from build123d import *

# Parameters (mm, degrees)
ESQUISSE1_R             = 1.5
ESQUISSE1_W             = 30
ESQUISSE1_H             = 6
BOSS_EXTRU_3_DEPTH      = 6
ESQUISSE4_W             = 6
ESQUISSE4_H             = 28
ESQUISSE4_H_2           = 85
ESQUISSE4_H_3           = 51
ESQUISSE4_H_4           = 21
ENL_V_MAT_EXTRU_2_DEPTH = 6
ESQUISSE5_R             = 1.5
ENL_V_MAT_EXTRU_3_DEPTH = 9
ENL_V_START             = -3
ESQUISSE6_R             = 1.5
ENL_V_MAT_EXTRU_6_DEPTH = 3
ESQUISSE7_W             = 20
ESQUISSE7_H             = 6
ENL_V_MAT_EXTRU_7_DEPTH = 10
ENL_V_MAT_EXTRU_8_DEPTH = 6
ESQUISSE9_R             = 1.5
ESQUISSE9_W             = 30
ESQUISSE9_H             = 6
ENL_V_MAT_EXTRU_9_DEPTH = 6


with BuildPart() as part:
    # Esquisse1 → Boss.-Extru.3 (new body)
    with BuildSketch(Plane.XY):
        Polygon((19.996437878, 165.487179487), (-0.003562122, 165.487179487), (-0.003562122, -184.512820513), (139.996437878, -184.512820513), (139.996437878, 165.487179487), (119.996437878, 165.487179487), (119.996437878, 105.487179487), (19.996437878, 105.487179487), align=None)
        with Locations((22.996437878, -25.512820513)):
            Circle(ESQUISSE1_R, mode=Mode.SUBTRACT)
        with Locations((69.996437878, -25.512820513)):
            Rectangle(ESQUISSE1_W, ESQUISSE1_H, mode=Mode.SUBTRACT)
        with Locations((116.996437878, -25.512820513)):
            Circle(ESQUISSE1_R, mode=Mode.SUBTRACT)
        with Locations((14.996437878, 162.487179487)):
            Circle(ESQUISSE1_R, mode=Mode.SUBTRACT)
        with Locations((58.496437878, 95.487179487)):
            Circle(ESQUISSE1_R, mode=Mode.SUBTRACT)
        with Locations((81.496437878, 95.487179487)):
            Circle(ESQUISSE1_R, mode=Mode.SUBTRACT)
        with Locations((124.996437878, 162.487179487)):
            Circle(ESQUISSE1_R, mode=Mode.SUBTRACT)
    extrude(amount=BOSS_EXTRU_3_DEPTH)

    # Esquisse4 → Enlèv. mat.-Extru.2 (cut)
    with BuildSketch(Plane.XY):
        with Locations((2.996437878, 151.487179487)):
            Rectangle(ESQUISSE4_W, ESQUISSE4_H)
        with Locations((2.996437878, 64.987179487)):
            Rectangle(ESQUISSE4_W, ESQUISSE4_H_2)
        with Locations((2.996437878, -33.012820513)):
            Rectangle(ESQUISSE4_W, ESQUISSE4_H_3)
        with Locations((136.996437878, -18.012820513)):
            Rectangle(ESQUISSE4_W, ESQUISSE4_H_4)
        with Locations((136.996437878, 64.987179487)):
            Rectangle(ESQUISSE4_W, ESQUISSE4_H_2)
        with Locations((136.996437878, 151.487179487)):
            Rectangle(ESQUISSE4_W, ESQUISSE4_H)
    extrude(amount=ENL_V_MAT_EXTRU_2_DEPTH, mode=Mode.SUBTRACT)

    # Esquisse5 → Enlèv. mat.-Extru.3 (cut)
    with BuildSketch(Plane(origin=(0, 0, 0), x_dir=(0, 0, -1), z_dir=(1, 0, 0))):
        with Locations(Location((-3, -30.012820513, 0), (0, 0, 270))):
            Circle(ESQUISSE5_R)
        with Locations((-3, -0.012820513)):
            Circle(ESQUISSE5_R)
        with Locations(Location((-3, 90.487179487, 0), (0, 0, 270))):
            Circle(ESQUISSE5_R)
        with Locations((-3, 120.487179487)):
            Circle(ESQUISSE5_R)
    extrude(amount=ENL_V_MAT_EXTRU_3_DEPTH, mode=Mode.SUBTRACT)

    # Esquisse6 → Enlèv. mat.-Extru.6 (cut)
    with BuildSketch(Plane(origin=(133.996437878, 0, 0), x_dir=(0, 0, -1), z_dir=(1, 0, 0)).offset(ENL_V_START)):
        with Locations(Location((-3, 90.487179487, 0), (0, 0, 270))):
            Circle(ESQUISSE6_R)
        with Locations(Location((-3, 44.987179487, 0), (0, 0, 90))):
            Circle(ESQUISSE6_R)
        with Locations((-3, 120.487179487)):
            Circle(ESQUISSE6_R)
    extrude(amount=ENL_V_MAT_EXTRU_6_DEPTH, mode=Mode.SUBTRACT)

    # Esquisse7 → Enlèv. mat.-Extru.7 (cut)
    with BuildSketch(Plane.XY):
        with Locations((129.996437878, -181.512820513)):
            Rectangle(ESQUISSE7_W, ESQUISSE7_H)
        with Locations((89.996437878, -181.512820513)):
            Rectangle(ESQUISSE7_W, ESQUISSE7_H)
    extrude(amount=ENL_V_MAT_EXTRU_7_DEPTH, mode=Mode.SUBTRACT)

    # Esquisse8 → Enlèv. mat.-Extru.8 (cut)
    with BuildSketch(Plane.XY.offset(6)):
        with BuildLine():
            Line((79.996437878, -178.512820513), (79.996437878, -113.512820513))
            ThreePointArc((79.996437878, -113.512820513), (42.996437878, -100.746283227), (5.996437878, -113.512820513))
            Line((5.996437878, -113.512820513), (5.996437878, -58.512820513))
            Line((5.996437878, -58.512820513), (-0.003562122, -58.512820513))
            Line((-0.003562122, -58.512820513), (-0.003562122, -184.512820513))
            Line((-0.003562122, -184.512820513), (79.996437878, -184.512820513))
            Line((79.996437878, -184.512820513), (79.996437878, -178.512820513))
        make_face()
    extrude(amount=-ENL_V_MAT_EXTRU_8_DEPTH, mode=Mode.SUBTRACT)

    # Esquisse9 → Enlèv. mat.-Extru.9 (cut)
    with BuildSketch(Plane.XY.offset(6)):
        with Locations((116.996437878, 30.487179487)):
            Circle(ESQUISSE9_R)
        with Locations((22.996437878, 30.487179487)):
            Circle(ESQUISSE9_R)
        with Locations((69.996437878, 30.487179487)):
            Rectangle(ESQUISSE9_W, ESQUISSE9_H)
    extrude(amount=-ENL_V_MAT_EXTRU_9_DEPTH, mode=Mode.SUBTRACT)


solid = part.part
Check sheet for the modelled part. Datum: model origin and axes. Units: mm. A direction names the side the tool comes from. Round coordinates to 2 decimals unless told otherwise and drop trailing zeros. Order: outer loops, then holes, each group sorted by start corner. A loop starts at its lowest first (then second) coordinate and runs counter-clockwise, first axis right, second up. Notation, with made-up numbers: M 20.5,86 L 28.5,86 A10 ccw 28.5,96 Z; hole C 44,19 d10. An arc over 180 degrees is marked long. One line per item, written item: value. Start each with the question number.
1. Section check A-A on x = 69.5. Enter the section's corners in (y, z).
2. Gauge pin test, flat ends, axial feed: P1, Ø1, axis at x = 26, z = 2.5, coming from the -Y side; P2, Ø1, axis at y = 68.5, z = 5.5, coming from the +X side; P3, Ø3, axis at x = 90, z = 4, coming from the -Y side; P4, Ø2.5, axis at x = 117, y = 30.49, coming from the -Z side. Record the tip position at first contact, or that the pin passes through.
3. Scan lines: line 1 along Y through (x, z) = (3.75, 3); line 2 along Y through (x, z) = (66, 5.4); line 3 along X through (y, z) = (133, 5.05). Record each from-to range of solid material in increasing order.
4. Release check for a two-part mould opening along Y. For faces 6 (the flat face through (137, -7.513, 3)), 7 (the flat face through (127, 165.487, 3)), 8 (the flat face through (19.996, 135, 3)) record: released by +Y, released by -Y, zero draft, split by the parting line, or undercut.
5. Section check C-C on x = 107.5. Enter the section's corners in (y, z), and give its area (3 significant figures).
6. Section check B-B on y = -70.5. Enter the section's corners in (x, z).
7. Section check D-D on z = 3. Give the number of separate pieces and of enclosed holes in the cut face, and give its area (3 significant figures).
8. Access from +Z, -Z, +X, -X, +Y, -Y to the whole of each face (thin tool, end or side, straight path). Record for faces 1 (the flat face through (137, 137.487, 3)), 2 (the flat face through (3, 107.487, 3)), 3 (the flat face through (54.996, 30, 3)), 4 (the flat face through (133.996, 64, 3)), 5 (the flat face through (71, 105.487, 3)).
Results found:
1. outline: M -106.92,0 L -28.51,0 L -28.51,6 L -106.92,6 Z; M -22.51,0 L 27.49,0 L 27.49,6 L -22.51,6 Z; M 33.49,0 L 105.49,0 L 105.49,6 L 33.49,6 Z
2. P1: y = -103.35
2. P2: x = 134
2. P3: y = -178.51
2. P4: through
3. line 1: -7.51 to -1.51, 1.49 to 22.49, 107.49 to 118.99, 121.99 to 137.49
3. line 2: -105.33 to -28.51, -22.51 to 27.49, 33.49 to 105.49
3. line 3: 0 to 20, 120 to 140
4. face 6: undercut
4. face 7: released by +Y
4. face 8: zero draft
5. outline: M -184.51,0 L 105.49,0 L 105.49,6 L -184.51,6 Z
5. area: 1,740 mm^2
6. outline: M 6,0 L 140,0 L 140,6 L 6,6 Z
7. separate pieces: 1
7. enclosed holes: 13
7. area: 33,800 mm^2
8. face 1: +Z, -Z, +X, +Y
8. face 2: +Z, -Z, -X
8. face 3: +Z, -Z
8. face 4: +Z, -Z, +X
8. face 5: +Z, -Z, +Y
